```python
from build123d import *

# Parameters (mm, degrees)
BOSS_EXTRUDE1_DEPTH     = 33
CUT_EXTRUDE1_DEPTH      = 83.954293528
CUT_EXTRUDE1_DEPTH_BACK = 12
SKETCH3_W               = 9.481209811
SKETCH3_H               = 17.021727652
CUT_EXTRUDE2_DEPTH      = 22
SKETCH6_W               = 39.175540074
SKETCH6_H               = 11.416045591
BOSS_EXTRUDE3_DEPTH     = 26
CUT_EXTRUDE3_DEPTH      = 26


with BuildPart() as part:
    # Sketch1 → Boss-Extrude1 (new body)
    with BuildSketch(Plane(origin=(0, 0, 0), x_dir=(1, 0, 0), z_dir=(0, 1, 0))):
        with BuildLine():
            Line((27.99701897, 26.104397373), (30.497019389, 26.104397373))
            Line((30.497019389, 26.104397373), (32.996926828, 26.125958592))
            Line((32.996926828, 26.125958592), (32.946330796, 31.992296402))
            ThreePointArc((32.946330796, 31.992296402), (34.614300355, 33.056919945), (35.86386473, 34.591238885))
            Line((35.86386473, 34.591238885), (40.431539769, 35.753760832))
            Line((40.431539769, 35.753760832), (43.136211097, 35.223788843))
            Line((43.136211097, 35.223788843), (43.274382132, 19.203600277))
            Line((43.274382132, 19.203600277), (48.774177579, 19.251034952))
            Line((48.774177579, 19.251034952), (48.43630867, 58.425118026))
            Line((48.43630867, 58.425118026), (42.936513223, 58.377683351))
            Line((42.936513223, 58.377683351), (43.088196039, 40.790876563))
            Line((43.088196039, 40.790876563), (40.395268448, 39.959225491))
            Line((40.395268448, 39.959225491), (35.888631414, 40.775372904))
            ThreePointArc((35.888631414, 40.775372904), (33.583892359, 43.097075019), (30.420151943, 43.929462788))
            ThreePointArc((30.420151943, 43.929462788), (27.263708108, 43.06982034), (24.979078258, 40.728327384))
            Line((24.979078258, 40.728327384), (20.479647685, 39.873342894))
            Line((20.479647685, 39.873342894), (17.779647685, 40.681737919))
            Line((17.779647685, 40.681737919), (17.779647685, 58.269198812))
            Line((17.779647685, 58.269198812), (12.279647685, 58.269198812))
            Line((12.279647685, 58.269198812), (12.279647685, 19.093658738))
            Line((12.279647685, 19.093658738), (17.779647685, 19.093658738))
            Line((17.779647685, 19.093658738), (17.779647685, 35.114443143))
            Line((17.779647685, 35.114443143), (20.479647685, 35.667721822))
            Line((20.479647685, 35.667721822), (25.057179, 34.544636961))
            ThreePointArc((25.057179, 34.544636961), (26.319929615, 33.021151936), (27.99701897, 31.970953369))
            Line((27.99701897, 31.970953369), (27.99701897, 26.104397373))
        make_face()
    extrude(amount=BOSS_EXTRUDE1_DEPTH)

    # Sketch2 → Cut-Extrude1 (cut, two sides: drawn at the far end of the back side and taken through both)
    with BuildSketch(Plane.XZ.offset(-CUT_EXTRUDE1_DEPTH_BACK)):
        with BuildLine():
            Line((20.479647685, -35.667721822), (17.779647685, -35.114443143))
            Line((17.779647685, -35.114443143), (17.779647685, -40.681737919))
            Line((17.779647685, -40.681737919), (20.479647685, -39.873342894))
            Line((20.479647685, -39.873342894), (24.979078258, -40.728327384))
            ThreePointArc((24.979078258, -40.728327384), (27.263708108, -43.06982034), (30.420151943, -43.929462788))
            ThreePointArc((30.420151943, -43.929462788), (33.576595778, -43.084424394), (35.888631414, -40.775372904))
            Line((35.888631414, -40.775372904), (40.395268448, -39.959225491))
            Line((40.395268448, -39.959225491), (43.088196039, -40.790876563))
            Line((43.088196039, -40.790876563), (43.136211097, -35.223788843))
            Line((43.136211097, -35.223788843), (40.431539769, -35.753760832))
            Line((40.431539769, -35.753760832), (35.86386473, -34.591238885))
            ThreePointArc((35.86386473, -34.591238885), (34.614300355, -33.056919945), (32.946330796, -31.992296402))
            Line((32.946330796, -31.992296402), (32.996926828, -26.125958592))
            Line((32.996926828, -26.125958592), (27.99701897, -26.104397373))
            Line((27.99701897, -26.104397373), (27.99701897, -31.970953369))
            ThreePointArc((27.99701897, -31.970953369), (26.319929615, -33.021151936), (25.057179, -34.544636961))
            Line((25.057179, -34.544636961), (20.479647685, -35.667721822))
        make_face()
    extrude(amount=CUT_EXTRUDE1_DEPTH + CUT_EXTRUDE1_DEPTH_BACK, mode=Mode.SUBTRACT)

    # Sketch3 → Cut-Extrude2 (cut)
    with BuildSketch(Plane.XY.offset(-26.104397373)):
        with Locations((32.737623876, 3.489136174)):
            Rectangle(SKETCH3_W, SKETCH3_H)
    extrude(amount=-CUT_EXTRUDE2_DEPTH, mode=Mode.SUBTRACT)

    # Sketch6 → Boss-Extrude3 (add)
    with BuildSketch(Plane(origin=(17.779647685, 0, 0), x_dir=(0, 0, -1), z_dir=(1, 0, 0))):
        with Locations((38.681428775, 27.291977205)):
            Rectangle(SKETCH6_W, SKETCH6_H)
    extrude(amount=BOSS_EXTRUDE3_DEPTH)

    # Sketch7 → Cut-Extrude3 (cut)
    with BuildSketch(Plane.XZ.offset(-21.583954409)):
        with BuildLine():
            Line((32.946330796, -31.992296402), (32.996926828, -26.125958592))
            Line((32.996926828, -26.125958592), (27.99701897, -26.104397373))
            Line((27.99701897, -26.104397373), (27.99701897, -31.970953369))
            ThreePointArc((27.99701897, -31.970953369), (22.888333328, -29.85486649), (17.779647685, -31.970953369))
            Line((17.779647685, -31.970953369), (17.779647685, -19.093658738))
            Line((17.779647685, -19.093658738), (43.274382132, -19.093658738))
            Line((43.274382132, -19.093658738), (43.779647685, -19.093658738))
            Line((43.779647685, -19.093658738), (43.779647685, -19.207958095))
            Line((43.779647685, -19.207958095), (43.274382132, -19.203600277))
            Line((43.274382132, -19.203600277), (43.164082095, -31.992296402))
            ThreePointArc((43.164082095, -31.992296402), (38.055206446, -29.876130819), (32.946330796, -31.992296402))
        make_face()
        with BuildLine():
            Line((43.205296614, -43.929694297), (42.937448882, -58.269198812))
            Line((42.937448882, -58.269198812), (17.779647685, -58.269198812))
            Line((17.779647685, -58.269198812), (17.779647685, -43.438467364))
            ThreePointArc((17.779647685, -43.438467364), (22.888333328, -45.554554244), (27.99701897, -43.438467364))
            ThreePointArc((27.99701897, -43.438467364), (29.185032105, -43.80020425), (30.420151943, -43.929462788))
            ThreePointArc((30.420151943, -43.929462788), (31.737082796, -43.800165691), (32.996926828, -43.395421786))
            ThreePointArc((32.996926828, -43.395421786), (37.990460261, -45.776780649), (43.205296614, -43.929694297))
        make_face()
    extrude(amount=-CUT_EXTRUDE3_DEPTH, mode=Mode.SUBTRACT)


solid = part.part
```
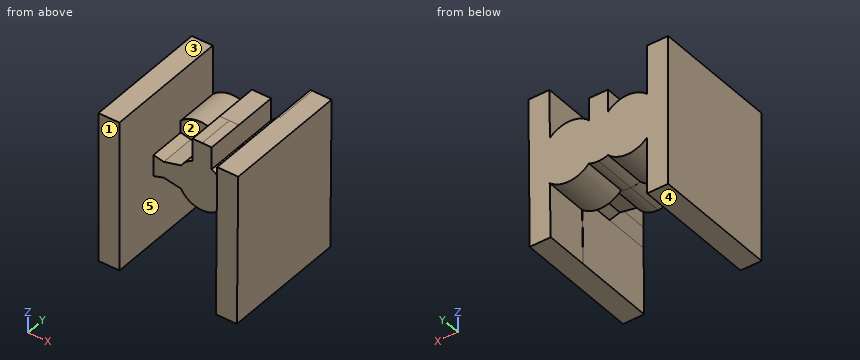
CAD build for the part. Positions are in the model's coordinates, mm. Face numbers are marked on the shaded views. A direction names the side the tool comes from. Give positions to 0.01 mm unless a question says otherwise; leave off trailing zeros. Order: outer loops, then holes, each group sorted by start corner. A loop starts at its lowest first (then second) coordinate and runs counter-clockwise, first axis right, second up.
(1) Saw through at C-C, the plane y = 26. Give the cut face in (x, z), then the cut area to 3 significant figures.
(2) Flat gauge pins, fed straight in: pin 1 (3 mm diameter, centred on x = 20.5, z = -33.5, fed in from -Y); pin 2 (19.5 mm diameter, centred on x = 28, z = -37, fed in from -Y); pin 3 (1.3 mm diameter, centred on x = 28.5, y = 19, fed in from +Z). Where does each tip first touch, or does it go through?
(3) Mould opens along Z. For the marked faces 3, 4 and 5 say: released by +Z, released by -Z, zero draft, split by the parting line, or undercut.
(4) Saw through at D-D, the plane x = 37.5. Give the cut face in (y, z).
(5) Drill centre lines: L1, parallel to Y at x = 31, z = -39; L2, parallel to Z at x = 17.5, y = 10; L3, parallel to X at y = 11.5, z = -48.5. Where is each one in solid material? Low to high.
(6) Saw through at B-B, the plane z = -24. Give the cut face in (x, y).
(7) Saw through at A-A, the plane y = 11. Give the cut face in (x, z).
(8) Tool access for the marked faces 1 and 2: list every direction of +Z, -Z, +X, -X, +Y, -Y with a clear straight run to the whole face (end or side of a thin tool).
Results found:
1. outline: (12.28, -58.27) - (17.78, -58.27) - (17.78, -43.44) arc R7.22 ccw to (28, -43.44) arc R6.5 ccw to (30.42, -43.93) arc R6.22 ccw to (33, -43.4) arc R7.23 ccw to (43.21, -43.93) - (42.94, -58.27) - (42.94, -58.38) - (48.44, -58.43) - (48.77, -19.25) - (43.27, -19.2) - (43.16, -31.99) arc R7.23 ccw to (32.95, -31.99) - (33, -26.13) - (28, -26.1) - (28, -31.97) arc R7.22 ccw to (17.78, -31.97) - (17.78, -19.09) - (12.28, -19.09) - close
1. area: 813 mm2
2. pin 1: stops at y = 21.58
2. pin 2: stops at y = 12
2. pin 3: stops at z = -26.1
3. face 3: released by +Z
3. face 4: released by -Z
3. face 5: zero draft
4. outline: (12, -40.48) - (21.58, -40.48) - (21.58, -45.73) - (33, -45.73) - (33, -29.9) - (21.58, -29.9) - (21.58, -35.01) - (12, -35.01) - close
5. L1: y = 12 to 33
5. L2: z = -58.27 to -19.09
5. L3: x = 12.28 to 17.78, 43.02 to 48.52
6. outline: (12.28, 0) - (17.78, 0) - (17.78, 33) - (12.28, 33) - close; (43.23, 0) - (48.73, 0) - (48.73, 33) - (43.23, 33) - close
7. outline: (12.28, -58.27) - (17.78, -58.27) - (17.78, -19.09) - (12.28, -19.09) - close; (42.94, -58.38) - (48.44, -58.43) - (48.77, -19.25) - (43.27, -19.2) - close
8. face 1: +Z, -Z, +X, -X, -Y
8. face 2: +Z, -Y
